Part model, mm, in its own coordinate system. A direction names the side the tool comes from. Round coordinates to 2 decimals unless told otherwise and drop trailing zeros. Loops run counter-clockwise (first coordinate to the right, second up) from the corner with the lowest first, then second, coordinate; pieces in that order, holes last. Notation, with made-up numbers: (72, 35) -> (76, 35) arc R37 cw to (76, 71) -> close; hole circle Ø1 at (53.5, 4.5). An arc over 180 degrees is marked (long way). Use a Markdown table: item, result. Add a question column.
Item 1: Flat gauge pins, fed straight in: pin 1 (2.5 mm diameter, centred on x = 0, y = 0, fed in from +Z); pin 2 (2.5 mm diameter, centred on x = 2, z = -1.5, fed in from -Y); pin 3 (1.1 mm diameter, centred on x = 1, z = -1.5, fed in from +Y). Where does each tip first touch, or does it go through?
Item 2: Probe line 1 (Z direction, x = 25, y = -2.75); line 2 (Z direction, x = 4, y = 2); line 3 (Y direction, x = 0, z = 0.8). List the from-to ranges inside material, lowest first. Write a range as [from, to].
Item 3: Cut at B-B, the plane x = 18.5. List the corners of the cut face in (y, z), plus the area to 3 significant figures.
Item 4: Two-plate mould, pull along Z, no slides. Class faces 4 (the face through (18, 0, -3.8)), 5 (the face through (28.5, 4.32, -4.31)), 6 (the face through (0, 2.85, -1)): pulls with the +Z half, pulls with the -Z half, needs draft (parallel to the pull), parting line crosses it, or undercut.
Item 5: Cut at C-C, the plane z = -5.75. List the corners of the cut face in (x, y), plus the area to 3 significant figures.
Item 6: Cut at D-D, the plane x = 3.5. List the corners of the cut face in (y, z), plus the area to 3 significant figures.
Item 7: Which spindle directions (+Z, -Z, +X, -X, +Y, -Y) get a long thin tool onto all of the face, cutting with end or side? Do faces 1 (the face through (12, 5.75, -4)), 2 (the face through (-1.216, 1.115, 0.69)), 3 (the face through (0, -2.85, -1)). Say none if no direction does.
Item 8: Cut at A-A, the plane y = 0. List the corners of the cut face in (x, z).
```python
from build123d import *

# Parameters (mm, degrees)
SKETCH121_R      = 5.7
SKETCH121_R_2    = 1.65
PAD123_DEPTH     = 1.4
PAD123_FACE3_R   = 5.7
PAD123_FACE3_R_2 = 1.65
PAD124_DEPTH     = 2.2
SKETCH122_W      = 27.339446
SKETCH122_H      = 5.7
POCKET083_DEPTH  = 2.2
SKETCH123_R      = 5.75
PAD125_DEPTH     = 1.6
PAD126_DEPTH     = 3
FILLET054_R      = 5
FILLET055_R      = 2
SKETCH125_R      = 1.65
POCKET084_DEPTH  = 5


with BuildPart() as part:
    # Sketch121 → Pad123 (new body)
    with BuildSketch(Plane.XY):
        Circle(SKETCH121_R)
        Circle(SKETCH121_R_2, mode=Mode.SUBTRACT)
    extrude(amount=PAD123_DEPTH)

    # Pad123 Face3 → Pad124 (add)
    with BuildSketch(Plane(origin=(0, 0, 0), x_dir=(0, -1, 0), z_dir=(0, 0, -1))):
        Circle(PAD123_FACE3_R)
        Circle(PAD123_FACE3_R_2, mode=Mode.SUBTRACT)
    extrude(amount=PAD124_DEPTH)

    # Sketch122 (on Face1 of Pad124) → Pocket083 (cut)
    with BuildSketch(Plane(origin=(0, 0, -2.2), x_dir=(1, 0, 0), z_dir=(0, 0, -1))):
        Rectangle(SKETCH122_W, SKETCH122_H)
    extrude(amount=-POCKET083_DEPTH, mode=Mode.SUBTRACT)

    # Sketch123 (on Face1 of Pocket083) → Pad125 (join)
    with BuildSketch(Plane(origin=(0, 0, -2.2), x_dir=(1, 0, 0), z_dir=(0, 0, -1))):
        Circle(SKETCH123_R)
    extrude(amount=PAD125_DEPTH)

    # Sketch124 (on Face3 of Pad125) → Pad126 (join)
    with BuildSketch(Plane(origin=(0, 0, -3.8), x_dir=(1, 0, 0), z_dir=(0, 0, -1))):
        with BuildLine():
            ThreePointArc((0, 5.75), (-5.75, 0), (0, -5.75))
            Line((0, -5.75), (30, -5.75))
            Line((30, 5.75), (30, -5.75))
            Line((0, 5.75), (30, 5.75))
        make_face()
    extrude(amount=PAD126_DEPTH)

    # Fillet054
    fillet054_edges = [part.edges().sort_by_distance(p)[0] for p in [
        (30, -5.75, -5.3),
        (30, 5.75, -5.3),
    ]]
    fillet(fillet054_edges, radius=FILLET054_R)

    # Fillet055
    fillet055_edges = [part.edges().sort_by_distance(p)[0] for p in [
        (28.535534, -4.285534, -6.8),
    ]]
    fillet(fillet055_edges, radius=FILLET055_R)

    # Sketch125 (on Face4 of Fillet055) → Pocket084 (cut)
    with BuildSketch(Plane.XY.offset(-3.8)):
        with Locations((25, 0)):
            Circle(SKETCH125_R)
    extrude(amount=-POCKET084_DEPTH, mode=Mode.SUBTRACT)


solid = part.part
```
A:
| question | item | result |
|---|---|---|
| 1 | pin 1 | stops at z = -2.2 |
| 1 | pin 2 | stops at y = -5.67 |
| 1 | pin 3 | stops at y = 5.68 |
| 2 | line 1 | z = [-6.8, -3.8] |
| 2 | line 2 | z = [-6.8, -2.2], [0, 1.4] |
| 2 | line 3 | y = [-5.7, -1.65], [1.65, 5.7] |
| 3 | outline | (-5.75, -4.8) arc R2 ccw to (-3.75, -6.8) -> (3.75, -6.8) arc R2 ccw to (5.75, -4.8) -> (5.75, -3.8) -> (-5.75, -3.8) -> close |
| 3 | area | 32.8 mm^2 |
| 4 | face 4 | pulls with the +Z half |
| 4 | face 5 | needs draft |
| 4 | face 6 | undercut |
| 5 | outline | (0, -5.51) -> (25, -5.51) arc R4.76 ccw to (29.76, -0.75) -> (29.76, 0.75) arc R4.76 ccw to (25, 5.51) -> (0, 5.51) arc R5.51 ccw to start; hole circle Ø3.3 at (25, 0) |
| 5 | area | 357 mm^2 |
| 6 | outline | (-5.75, -4.8) arc R2 ccw to (-3.75, -6.8) -> (3.75, -6.8) arc R2 ccw to (5.75, -4.8) -> (5.75, -3.8) -> (4.56, -3.8) -> (4.56, -2.2) -> (4.5, -2.2) -> (4.5, 1.4) -> (-4.5, 1.4) -> (-4.5, -2.2) -> (-4.56, -2.2) -> (-4.56, -3.8) -> (-5.75, -3.8) -> close; hole (-2.85, -2.2) -> (2.85, -2.2) -> (2.85, 0) -> (-2.85, 0) -> close |
| 6 | area | 67.2 mm^2 |
| 7 | face 1 | +Z, -Z, +X, -X, +Y |
| 7 | face 2 | +Z |
| 7 | face 3 | +X, -X |
| 8 | outline | (-5.75, -4.8) arc R2 ccw to (-3.75, -6.8) -> (23.35, -6.8) -> (23.35, -3.8) -> (5.75, -3.8) -> (5.75, -2.2) -> (-5.75, -2.2) -> close; (-5.7, 0) -> (-1.65, 0) -> (-1.65, 1.4) -> (-5.7, 1.4) -> close; (1.65, 0) -> (5.7, 0) -> (5.7, 1.4) -> (1.65, 1.4) -> close; (26.65, -6.8) -> (28, -6.8) arc R2 ccw to (30, -4.8) -> (30, -3.8) -> (26.65, -3.8) -> close |
